```python
from build123d import *

# Parameters (mm, degrees)
F1_DEPTH  = 55
F2_R      = 3
F3_DEPTH  = 55.001
F4_R      = 18
F5_DEPTH  = 4.7
F6_R      = 9
F7_DEPTH  = 4
F9_DEPTH  = 55.001
F10_R     = 3
F10_R_2   = 4.5
F11_DEPTH = 55.001
F13_DEPTH = 10
F15_DEPTH = 5.2
F16_W     = 9
F16_H     = 9
F17_DEPTH = 2.7


with BuildPart() as f1:
    # F0 (on Top) → F1 (new body)
    with BuildSketch(Plane.XY):
        Polygon((61.611576, 15.259703), (-56.888424, 15.259703), (-56.888424, -133.240297), (-7.388424, -133.240297), (-7.388424, -107.740297), (61.611576, -107.740297), align=None)
    extrude(amount=F1_DEPTH)

    # F2 (on face) → F3 (cut, through all)
    with BuildSketch(Plane.XY.offset(55)):
        with Locations((-47.888424, -98.740297)):
            Circle(F2_R)
        with Locations((52.611576, -98.740297)):
            Circle(F2_R)
        with BuildLine():
            ThreePointArc((49.611576, 6.259703), (52.611576, 3.259703), (55.611576, 6.259703))
            ThreePointArc((55.611576, 6.259703), (52.611576, 9.259703), (49.611576, 6.259703))
        make_face()
        with Locations((-47.888424, 6.259703)):
            Circle(F2_R)
    extrude(amount=-F3_DEPTH, mode=Mode.SUBTRACT)

    # F4 (on face) → F5 (join)
    with BuildSketch(Plane.XY.offset(55)):
        with Locations((-20.888424, -71.240297)):
            Circle(F4_R)
    extrude(amount=F5_DEPTH)

    # F6 (on face) → F7 (join)
    with BuildSketch(Plane.XY.offset(55)):
        with Locations((18.111576, -71.240297)):
            Circle(F6_R)
        with Locations((43.611576, -71.240297)):
            Circle(F6_R)
    extrude(amount=F7_DEPTH)

    # F8 (on face) → F9 (cut, through all)
    with BuildSketch(Plane.XY.offset(55)):
        with BuildLine():
            Line((12.111576, -40.240297), (12.111576, -22.240297))
            ThreePointArc((12.111576, -22.240297), (9.111576, -19.240297), (6.111576, -22.240297))
            Line((6.111576, -22.240297), (6.111576, -40.240297))
            ThreePointArc((6.111576, -40.240297), (9.111576, -43.240297), (12.111576, -40.240297))
        make_face()
    extrude(amount=-F9_DEPTH, mode=Mode.SUBTRACT)

    # F10 (on face) → F11 (cut, through all)
    with BuildSketch(Plane.XY.offset(55)):
        with Locations((33.111576, -36.740297)):
            Circle(F10_R)
        with Locations((43.111576, -36.740297)):
            Circle(F10_R_2)
    extrude(amount=-F11_DEPTH, mode=Mode.SUBTRACT)

    # F12 (on face) → F13 (cut)
    with BuildSketch(Plane.XY.offset(55)):
        with BuildLine():
            Line((-23.888424, -2.740297), (-47.888424, -2.740297))
            Line((-47.888424, -2.740297), (-47.888424, -26.740297))
            Line((-47.888424, -26.740297), (-40.388424, -26.740297))
            Line((-40.388424, -26.740297), (-40.388424, -10.240297))
            Line((-40.388424, -10.240297), (-23.888424, -10.240297))
            ThreePointArc((-23.888424, -10.240297), (-20.138424, -6.490297), (-23.888424, -2.740297))
        make_face()
    extrude(amount=-F13_DEPTH, mode=Mode.SUBTRACT)

    # F14 (on face) → F15 (join)
    with BuildSketch(Plane.XY.offset(55)):
        with BuildLine():
            ThreePointArc((-20.888424, -33.740297), (-23.009744, -38.861618), (-17.888424, -36.740297))
            ThreePointArc((-17.888424, -36.740297), (-18.767104, -34.618977), (-20.888424, -33.740297))
        make_face()
    extrude(amount=F15_DEPTH)

    # F16 (on face) → F17 (join)
    with BuildSketch(Plane.XY.offset(55)):
        with Locations((-47.888424, -121.240297)):
            Rectangle(F16_W, F16_H)
        with Locations((-31.388424, -121.240297)):
            Rectangle(F16_W, F16_H)
        with Locations((-14.888424, -121.240297)):
            Rectangle(F16_W, F16_H)
    extrude(amount=F17_DEPTH)


solid = f1.part
```
Input: part model. Units: mm. Frame: model coordinates. A direction names the side the tool comes from. Give positions to 0.01 mm unless a question says otherwise; leave off trailing zeros. Order: outer loops, then holes, each group sorted by start corner. A loop starts at its lowest first (then second) coordinate and runs counter-clockwise, first axis right, second up. Notation, with made-up numbers: M -15.75,47.5 L 0.25,47.5 A8 cw 0.25,53.5 Z; hole C -32,78 d2. An arc over 180 degrees is marked long. Return JSON: item names as keys, results as strings.
Item 1: Ray query, probe 1 along X at (y, z) = (-7, 45.5); probe 2 along Y at (x, z) = (54.5, 36.5); probe 3 along Z at (x, y) = (-2.5, -57). Return the intervals inside material, ascending.
Solutions:
{"probe 1": "-56.89 to -47.89, -20.17 to 61.61", "probe 2": "-107.74 to -101.07, -96.41 to 3.93, 8.59 to 15.26", "probe 3": "0 to 55"}
Item 2: Access query for faces 1 (the flat face through (18, -71, 59)), 2 (the cylindrical face through (55.473, -97.839, 27.885)), 3 (the cylindrical face through (-20.14, -6.57, 50.07)), 4 (the flat face through (-21, -71, 59.7)). Directions: +Z, -Z, +X, -X, +Y, -Y. A direction counts if a zero-diameter tool reaches every point of the face in a straight line with its end or side. Return the directions, or none.
Solutions:
{"face 1": "+Z, +X, +Y, -Y", "face 2": "+Z, -Z", "face 3": "+Z", "face 4": "+Z, +X, -X, -Y"}
Item 3: Cut plane A-A (x = 44). Return loops of the section in (y, z).
Solutions:
{"outline": "M -107.74,0 L -41.15,0 L -41.15,55 L -62.25,55 L -62.25,59 L -80.23,59 L -80.23,55 L -107.74,55 Z; M -32.33,0 L 15.26,0 L 15.26,55 L -32.33,55 Z"}
Item 4: Cut plane C-C (z = 30). Return loops of the section in (x, y), then the cut area to 3 significant figures.
Solutions:
{"outline": "M -56.89,-133.24 L -7.39,-133.24 L -7.39,-107.74 L 61.61,-107.74 L 61.61,15.26 L -56.89,15.26 Z; hole C -47.89,-98.74 d6; hole C -47.89,6.26 d6; hole M 6.11,-40.24 A3 ccw 12.11,-40.24 L 12.11,-22.24 A3 ccw 6.11,-22.24 Z; hole C 33.11,-36.74 d6; hole C 43.11,-36.74 d9; hole C 52.61,-98.74 d6; hole C 52.61,6.26 d6", "area": "15,500 mm^2"}
Item 5: Cut plane B-B (z = 51). State how many separate pieces and enclosed holes the cut face has, then the cut area to 3 significant figures.
Solutions:
{"separate pieces": "1", "enclosed holes": "8", "area": "15,200 mm^2"}
Item 6: Cut plane D-D (y = -68). Return loops of the section in (x, z).
Solutions:
{"outline": "M -56.89,0 L 61.61,0 L 61.61,55 L 52.01,55 L 52.01,59 L 35.22,59 L 35.22,55 L 26.51,55 L 26.51,59 L 9.72,59 L 9.72,55 L -3.18,55 L -3.18,59.7 L -38.59,59.7 L -38.59,55 L -56.89,55 Z"}
Item 7: First-contact query: P1, Ø2.5, axis at x = -32, y = -123.5, coming from the +Z side; P2, Ø3, axis at x = -47, z = 57, coming from the +Y side; P3, Ø1.5, axis at x = 25, z = 13.5, coming from the -Y side; P4, Ø8, axis at x = 43.11, y = -36.74, coming from the -Z side. Flat tips, straight axial feed; report the tip coordinate or a pass-through.
Solutions:
{"P1": "z = 57.7", "P2": "y = -116.74", "P3": "y = -107.74", "P4": "through"}
Item 8: Pull-direction query (X, two-part tool) for faces 5 (the flat face through (2, -58, 0)), 6 (the flat face through (-37, -9, 45)), 7 (the flat face through (-7.388, -121, 27)), 8 (the cylindrical face through (55.473, 7.161, 27.885)); classes: +X half, -X half, draft (parallel to the pull), parting line (faces both ways), or undercut.
Solutions:
{"face 5": "draft", "face 6": "undercut", "face 7": "+X half", "face 8": "undercut"}
